Geometry check sheet. Reference: the model listing, model coordinates, mm. A direction names the side the tool comes from. Give positions to 0.01 mm unless a question says otherwise; leave off trailing zeros. Write each loop counter-clockwise with the first axis right and the second up, starting at its lowest first coordinate (ties: lowest second). Pieces come first, ordered by that corner, then holes. Notation, with made-up numbers: (70, 67) - (93, 67) arc R25 cw to (93, 86) - close; hole circle Ø7 at (53, 7). An arc over 180 degrees is marked (long way). Write item = value, one per line. Start each with the question number.
(1) Section check C-C, the plane x = -20.5. Enter the section's corners in (y, z).
(2) Draft check along Y on faces 1 (the flat face through (-1, -36.5, 2)), 2 (the flat face through (-1, 36.5, 2)), 3 (the flat face through (-50, -1, 1)), 4 (the flat face through (-9, 5, 3)). Enter one of: pulls with the +Y half, pulls with the -Y half, needs draft (parallel to the pull), parting line crosses it, or undercut.
(3) Section check B-B, the plane z = 2.25. Enter the section's corners in (x, y).
(4) Section check D-D, the plane x = -36. Enter the section's corners in (y, z).
(5) Access from +Z, -Z, +X, -X, +Y, -Y to the whole of each face (thin tool, end or side, straight path). Record for faces 5 (the flat face through (-39, 0, 1.5)), 6 (the flat face through (50, -1, 1)), 7 (the flat face through (-23, 30, 3)), 8 (the flat face through (20, 15, 3)).
(6) Depth check by flat-ended pin: pin 1 Ø2.5 at (y, z) = (3.5, 3.5) entering from -X; pin 2 Ø6 at (x, y) = (12, 9) entering from +Z. Enter the tip coordinate at first touch or a pass-through.
(7) Section check A-A, the plane y = -2. Enter the section's corners in (x, z), plus the area to 3 significant figures.
(8) Thickness scan on L1, parallel to X at y = 21.5, z = 4.45; L2, parallel to Y at x = 41.5, z = 1.65; L3, parallel to Y at x = 14, z = 4.7. Record the ranges inside material, lowest first.
```python
from build123d import *

# Parameters (mm, degrees)
SKETCH_W        = 100
SKETCH_H        = 73
PAD_DEPTH       = 5
SKETCH001_W     = 22.5
SKETCH001_H     = 10
POCKET_DEPTH    = 3.5
SKETCH002_W     = 10
SKETCH002_H     = 60
POCKET001_DEPTH = 5
SKETCH003_W     = 67.5
SKETCH003_H     = 10
POCKET002_DEPTH = 3.5
SKETCH004_W     = 20
SKETCH004_H     = 20
POCKET003_DEPTH = 3.5


with BuildPart() as part:
    # Sketch → Pad (new body)
    with BuildSketch(Plane.XY):
        Rectangle(SKETCH_W, SKETCH_H)
    extrude(amount=PAD_DEPTH)

    # Sketch001 (on Face6 of Pad) → Pocket (cut)
    with BuildSketch(Plane.XY.offset(5)):
        with Locations((-38.75, 0)):
            Rectangle(SKETCH001_W, SKETCH001_H)
    extrude(amount=-POCKET_DEPTH, mode=Mode.SUBTRACT)

    # Sketch002 (on Face5 of Pocket) → Pocket001 (cut)
    with BuildSketch(Plane.XY.offset(5)):
        with Locations((-22.5, 0)):
            Rectangle(SKETCH002_W, SKETCH002_H)
    extrude(amount=-POCKET001_DEPTH, mode=Mode.SUBTRACT)

    # Sketch003 (on Face5 of Pocket001) → Pocket002 (cut)
    with BuildSketch(Plane.XY.offset(5)):
        with Locations((16.25, 0)):
            Rectangle(SKETCH003_W, SKETCH003_H)
    extrude(amount=-POCKET002_DEPTH, mode=Mode.SUBTRACT)

    # Sketch004 (on Face5 of Pocket002) → Pocket003 (cut)
    with BuildSketch(Plane.XY.offset(5)):
        with Locations((10, 15)):
            Rectangle(SKETCH004_W, SKETCH004_H)
    extrude(amount=-POCKET003_DEPTH, mode=Mode.SUBTRACT)


solid = part.part
```
Model answer:
q1.outline = (-36.5, 0) - (-30, 0) - (-30, 5) - (-36.5, 5) - close; (30, 0) - (36.5, 0) - (36.5, 5) - (30, 5) - close
q2.face_1 = pulls with the -Y half
q2.face_2 = pulls with the +Y half
q2.face_3 = needs draft
q2.face_4 = undercut
q3.outline = (-50, -36.5) - (50, -36.5) - (50, -5) - (-17.5, -5) - (-17.5, -30) - (-27.5, -30) - (-27.5, -5) - (-50, -5) - close; (-50, 5) - (-27.5, 5) - (-27.5, 30) - (-17.5, 30) - (-17.5, 5) - (0, 5) - (0, 25) - (20, 25) - (20, 5) - (50, 5) - (50, 36.5) - (-50, 36.5) - close
q4.outline = (-36.5, 0) - (36.5, 0) - (36.5, 5) - (5, 5) - (5, 1.5) - (-5, 1.5) - (-5, 5) - (-36.5, 5) - close
q5.face_5 = +Z, +X, -X
q5.face_6 = +Z, -Z, +X, +Y, -Y
q5.face_7 = +Z, -Z
q5.face_8 = +Z
q6.pin_1 = through
q6.pin_2 = 1.5
q7.outline = (-50, 0) - (-27.5, 0) - (-27.5, 1.5) - (-50, 1.5) - close; (-17.5, 0) - (50, 0) - (50, 1.5) - (-17.5, 1.5) - close
q7.area = 135 mm²
q8.L1 = -50 to -27.5, -17.5 to 0, 20 to 50
q8.L2 = -36.5 to -5, 5 to 36.5
q8.L3 = -36.5 to -5, 25 to 36.5
